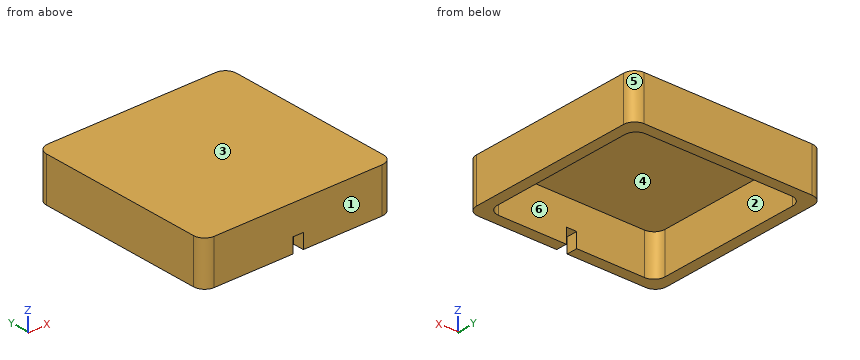
```python
from build123d import *

# Parameters (mm, degrees)
BOSS_EXTRUDE1_OUTLINE_W = 43.688
BOSS_EXTRUDE1_OUTLINE_H = 43.688
BOSS_EXTRUDE1_DEPTH     = 10.16
CUT_EXTRUDE2_DEPTH      = 9.398
SKETCH3_W               = 2.4
SKETCH3_H               = 3.4
CUT_EXTRUDE3_DEPTH      = 9.398
FILLET1_R               = 2.54
FILLET2_R               = 2.54


# Read off the part's stored shape, not the designer's step: Boss-Extrude1
with BuildPart() as part:
    # Boss-Extrude1 outline → Boss-Extrude1 (new body)
    with BuildSketch(Plane.XY):
        Rectangle(BOSS_EXTRUDE1_OUTLINE_W, BOSS_EXTRUDE1_OUTLINE_H)
    extrude(amount=BOSS_EXTRUDE1_DEPTH)

    # Sketch4 → Cut-Extrude2 (cut)
    with BuildSketch(Plane(origin=(0, 0, 0), x_dir=(-1, 0, 0), z_dir=(0, 0, -1))):
        Polygon((-19.304, 19.304), (0, 0), (19.304, 19.304), align=None)
        Polygon((-19.304, 19.304), (-19.304, -19.304), (0, 0), align=None)
        Polygon((19.304, 19.304), (0, 0), (19.304, -19.304), align=None)
        Polygon((0, 0), (-19.304, -19.304), (19.304, -19.304), align=None)
    extrude(amount=-CUT_EXTRUDE2_DEPTH, mode=Mode.SUBTRACT)

    # Sketch3 → Cut-Extrude3 (cut)
    with BuildSketch(Plane.XZ.offset(21.844)):
        with Locations((0, 1.7)):
            Rectangle(SKETCH3_W, SKETCH3_H)
    extrude(amount=-CUT_EXTRUDE3_DEPTH, mode=Mode.SUBTRACT)

    # Fillet1
    fillet1_edges = [part.edges().sort_by_distance(p)[0] for p in [
        (21.844, -21.844, 5.08),
        (-21.844, -21.844, 5.08),
        (-21.844, 21.844, 5.08),
        (21.844, 21.844, 5.08),
    ]]
    fillet(fillet1_edges, radius=FILLET1_R)

    # Fillet2
    fillet2_edges = [part.edges().sort_by_distance(p)[0] for p in [
        (19.304, 19.304, 4.699),
        (-19.304, 19.304, 4.699),
        (-19.304, -19.304, 4.699),
        (19.304, -19.304, 4.699),
    ]]
    fillet(fillet2_edges, radius=FILLET2_R)


solid = part.part
```
CAD build for the part. Positions are in the model's coordinates, mm. Face numbers are marked on the shaded views. A direction names the side the tool comes from. Coordinates: 2 decimals unless noted, no trailing zeros. Order: outer loops, then holes, each group sorted by start corner. A loop starts at its lowest first (then second) coordinate and runs counter-clockwise, first axis right, second up. Notation, with made-up numbers: (22.5, 24.25) - (38.5, 24.25) arc R23 ccw to (38.5, 48.25) - close; hole circle Ø10 at (67.25, -19.75). An arc over 180 degrees is marked (long way). Answer in a Markdown table with one row per item.
1. Slice it at B-B, the plane x = 7. List the corners of the cut face in (y, z).
Answer:
| item | result |
|---|---|
| outline | (-21.84, 0) - (-19.3, 0) - (-19.3, 9.4) - (19.3, 9.4) - (19.3, 0) - (21.84, 0) - (21.84, 10.16) - (-21.84, 10.16) - close |
2. Slice it at D-D, the plane z = 0.75. List the corners of the cut face in (x, y), then the cut area to 3 significant figures.
Answer:
| item | result |
|---|---|
| outline | (-21.84, -19.3) arc R2.54 ccw to (-19.3, -21.84) - (-1.2, -21.84) - (-1.2, -19.3) - (-16.76, -19.3) arc R2.54 cw to (-19.3, -16.76) - (-19.3, 16.76) arc R2.54 cw to (-16.76, 19.3) - (16.76, 19.3) arc R2.54 cw to (19.3, 16.76) - (19.3, -16.76) arc R2.54 cw to (16.76, -19.3) - (1.2, -19.3) - (1.2, -21.84) - (19.3, -21.84) arc R2.54 ccw to (21.84, -19.3) - (21.84, 19.3) arc R2.54 ccw to (19.3, 21.84) - (-19.3, 21.84) arc R2.54 ccw to (-21.84, 19.3) - close |
| area | 412 mm² |
3. Slice it at A-A, the plane z = 6. List the corners of the cut face in (x, y), then the cut area to 3 significant figures.
Answer:
| item | result |
|---|---|
| outline | (-21.84, -19.3) arc R2.54 ccw to (-19.3, -21.84) - (19.3, -21.84) arc R2.54 ccw to (21.84, -19.3) - (21.84, 19.3) arc R2.54 ccw to (19.3, 21.84) - (-19.3, 21.84) arc R2.54 ccw to (-21.84, 19.3) - close; hole (-19.3, -16.76) arc R2.54 ccw to (-16.76, -19.3) - (16.76, -19.3) arc R2.54 ccw to (19.3, -16.76) - (19.3, 16.76) arc R2.54 ccw to (16.76, 19.3) - (-16.76, 19.3) arc R2.54 ccw to (-19.3, 16.76) - close |
| area | 418 mm² |
4. Pull direction Y, two halves, no side cores. Call the marked faces 3, 4, 5 and 6: +Y half, -Y half, draft (parallel to the pull), parting line (faces both ways), or undercut.
Answer:
| item | result |
|---|---|
| face 3 | draft |
| face 4 | undercut |
| face 5 | +Y half |
| face 6 | undercut |
5. Drill centre lines: L1, parallel to X at y = -1.5, z = 5.75; L2, parallel to Y at x = 19.5, z = 6.5. Where is each one in solid material? Low to high. Write a range as from..to.
Answer:
| item | result |
|---|---|
| L1 | -21.84..-19.3, 19.3..21.84 |
| L2 | -21.84..21.84 |
6. 3-axis set-ups, long thin cutter, end or side, ignore diameter. For the marked faces 1 and 2: which of +Z, -Z, +X, -X, +Y, -Y reach the whole face in a straight line?
Answer:
| item | result |
|---|---|
| face 1 | +Z, -Z, +X, -X, -Y |
| face 2 | -Z |
7. Flat gauge pins, fed straight in: P1, Ø2, axis at y = -20.5, z = 1.5, coming from the +X side; P2, Ø2, axis at x = -5, y = -8.5, coming from the -Z side. Where does each tip first touch, or does it go through?
Answer:
| item | result |
|---|---|
| P1 | x = 21.84 |
| P2 | z = 9.4 |
